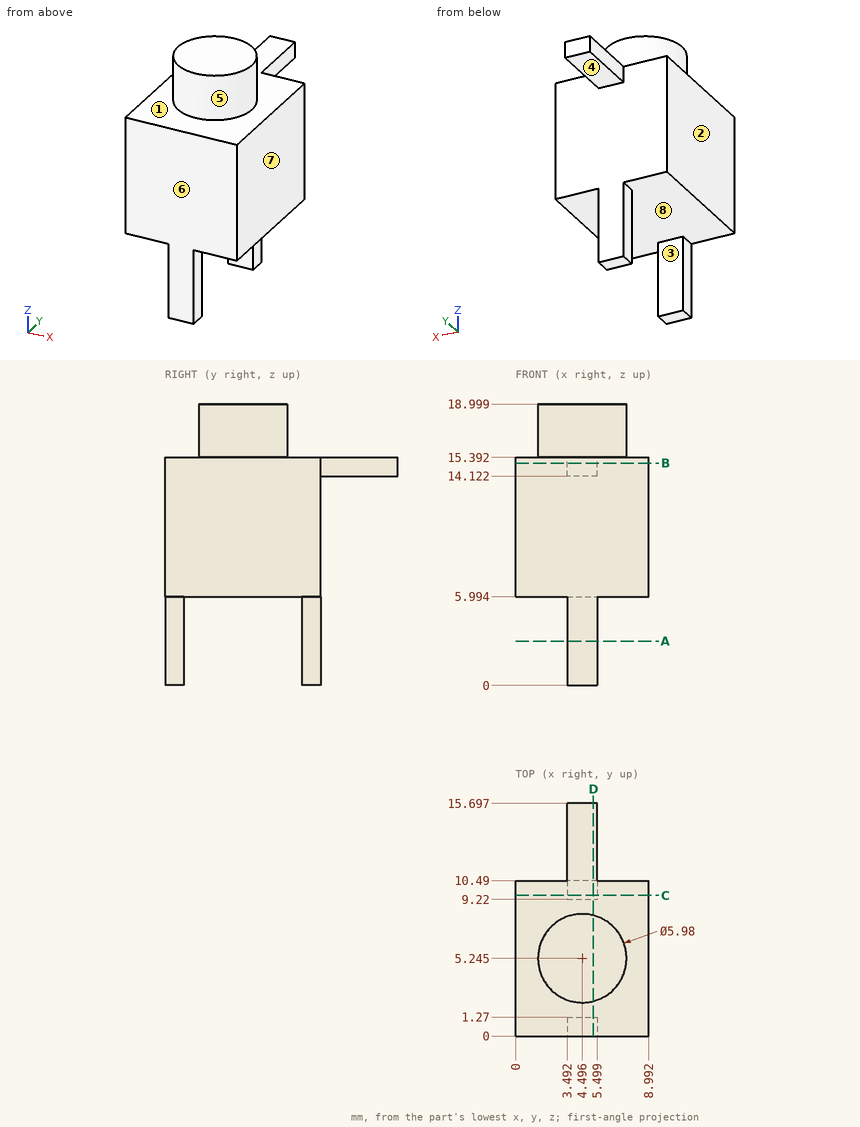
Could you check a few things on this drawing? It's one solid part, dimensions in mm from its lowest x, y, z. A direction names the side the tool comes from. Give positions to 0.01 mm unless a question says otherwise; leave off trailing zeros. Write each loop counter-clockwise with the first axis right and the second up, starting at its lowest first coordinate (ties: lowest second). Pieces come first, ordered by that corner, then holes. Notation, with made-up numbers: (55.5, 81) - (105.5, 81) arc R20 ccw to (105.5, 98) - close; hole circle Ø3 at (61.25, 24). An arc over 180 degrees is marked (long way). Use CSV: the item, a comma, the result in double quotes. Start each with the question number.
Item 1: If I drill on line 1 along Y through (x, z) = (1.5, 6.75); line 2 along Z through (x, y) = (6.5, 5.5) (1 decimal); line 3 along Z through (x, y) = (7.25, 2.75) (1 decimal), over which ranges is the centre line in solid material (lowest first)?
Item 2: I'm going to push flat-ended pins straight in: pin 1 (2 mm diameter, centred on x = 1.5, z = 13, fed in from -Y); pin 2 (1.4 mm diameter, centred on y = 0.5, z = 4, fed in from +X); pin 3 (2 mm diameter, centred on x = 2, y = 2, fed in from +Z); pin 4 (2 mm diameter, centred on x = 4.5, z = 2.5, fed in from +Y). Where does each tip first touch, or does it pass through?
Item 3: I want a section at C-C, the plane y = 9.5. Please give me the cut outline in (x, z) (1 decimal).
Item 4: I want a section at A-A, the plane z = 3. Please give me the cut outline in (x, y).
Item 5: I want a section at B-B, the plane z = 15. Please give me the cut outline in (x, y), then the cut area to 3 significant figures.
Item 6: For the marked faces 1, 2, 3 and 4, which set-ups out of +Z, -Z, +X, -X, +Y, -Y let a thin tool reach every point of the face, with its end or its side?
Item 7: I want a section at D-D, the plane x = 5.25. Please give me the cut outline in (y, z) (1 decimal), then the cut area to 3 significant figures.
Item 8: If we mould it in two halves opening along Y, with no side actions, what happens to the marked faces 5, 6, 7 and 8? For each: pulls with the +Y half, pulls with the -Y half, needs draft (parallel to the pull), parting line crosses it, or undercut.
Findings:
1,line 1,"y = 0 to 10.49"
1,line 2,"z = 6 to 19"
1,line 3,"z = 6 to 15.4"
2,pin 1,"stops at y = 0"
2,pin 2,"stops at x = 5.5"
2,pin 3,"stops at z = 15.39"
2,pin 4,"stops at y = 10.49"
3,outline,"(0, 6) - (3.5, 6) - (3.5, 0) - (5.5, 0) - (5.5, 6) - (9, 6) - (9, 15.4) - (0, 15.4) - close"
4,outline,"(3.49, 0) - (5.5, 0) - (5.5, 1.27) - (3.49, 1.27) - close; (3.49, 9.22) - (5.5, 9.22) - (5.5, 10.49) - (3.49, 10.49) - close"
5,outline,"(0, 0) - (8.99, 0) - (8.99, 10.49) - (5.5, 10.49) - (5.5, 15.7) - (3.49, 15.7) - (3.49, 10.49) - (0, 10.49) - close"
5,area,"105 mm2"
6,face 1,"+Z"
6,face 2,"+Z, -Z, -X, +Y, -Y"
6,face 3,"-Z, +X, -X"
6,face 4,"-Z, +X, -X, +Y"
7,outline,"(0, 0) - (1.3, 0) - (1.3, 6) - (9.2, 6) - (9.2, 0) - (10.5, 0) - (10.5, 14.1) - (15.7, 14.1) - (15.7, 15.4) - (8.1, 15.4) - (8.1, 19) - (2.4, 19) - (2.4, 15.4) - (0, 15.4) - close"
7,area,"141 mm2"
8,face 5,"parting line crosses it"
8,face 6,"pulls with the -Y half"
8,face 7,"needs draft"
8,face 8,"undercut"
